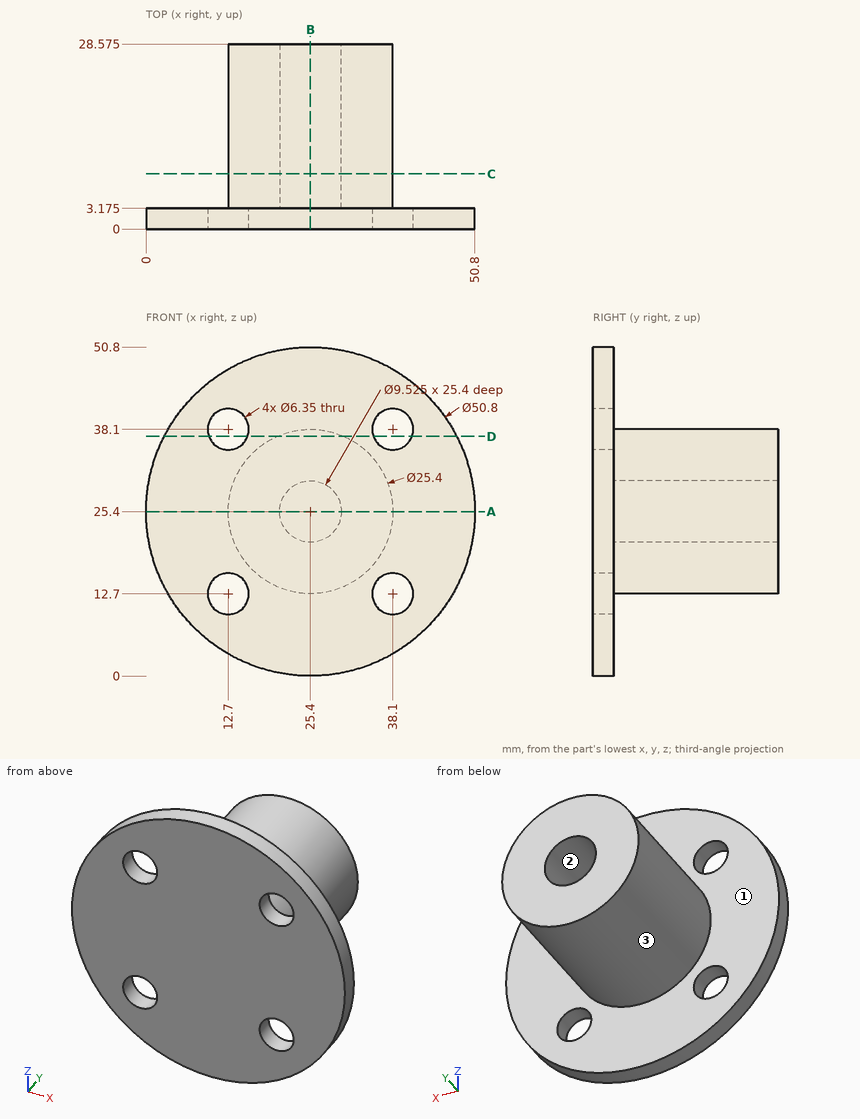
Drawing for the job (mm, zero at the part's lowest x, y, z). Give positions to 0.01 mm unless a question says otherwise; leave off trailing zeros. Order: outer loops, then holes, each group sorted by start corner. A loop starts at its lowest first (then second) coordinate and runs counter-clockwise, first axis right, second up. Notation, with made-up numbers: M -10,14 L 12,14 A17 ccw 12,44 Z; hole C -8,40 d10. An arc over 180 degrees is marked long. Put each result on its own line as item: value.
Item 1: Probe line 1 (X direction, y = 11, z = 25.4); line 2 (Z direction, x = 11, y = 1.5); line 3 (Z direction, x = 12.7, y = 1) (3 decimals). List the from-to ranges inside material, lowest first. Write a range as [from, to].
From the geometry:
line 1: x = [12.7, 20.64], [30.16, 38.1]
line 2: z = [4.48, 10.02], [15.38, 35.42], [40.78, 46.32]
line 3: z = [3.403, 9.525], [15.875, 34.925], [41.275, 47.397]
Item 2: Flat gauge pins, fed straight in: pin 1 Ø4 at (x, z) = (10.5, 33.5) entering from +Y (3 decimals); pin 2 Ø12 at (x, y) = (12.5, 16.5) entering from -Z; pin 3 Ø1 at (x, y) = (17.5, 23.5) entering from +Z. Where does each tip first touch, or does it go through?
From the geometry:
pin 1: stops at y = 3.175
pin 2: stops at z = 14.74
pin 3: stops at z = 35.72
Item 3: Slice it at B-B, the plane x = 25.4. Write the cut outline in (y, z) (1 decimal), plus the area to 3 significant figures.
From the geometry:
outline: M 0,0 L 3.2,0 L 3.2,12.7 L 28.6,12.7 L 28.6,20.6 L 3.2,20.6 L 3.2,30.2 L 28.6,30.2 L 28.6,38.1 L 3.2,38.1 L 3.2,50.8 L 0,50.8 Z
area: 565 mm2
Item 4: Slice it at C-C, the plane y = 8.5. Write the cut outline in (x, z) (1 decimal), plus the area to 3 significant figures.
From the geometry:
outline: C 25.4,25.4 d25.4; hole C 25.4,25.4 d9.5
area: 435 mm2
Item 5: Two-plate mould, pull along X, no slides. Class the marked faces 1, 2 and 3: +X half, -X half, draft (parallel to the pull), parting line (faces both ways), or undercut.
From the geometry:
face 1: draft
face 2: undercut
face 3: parting line
Item 6: Slice it at D-D, the plane z = 37. Write the cut outline in (x, y) (3 decimals), plus the area to 3 significant figures.
From the geometry:
outline: M 2.804,0 L 9.722,0 L 9.722,3.175 L 2.804,3.175 Z; M 15.678,0 L 35.122,0 L 35.122,3.175 L 30.57,3.175 L 30.57,28.575 L 20.23,28.575 L 20.23,3.175 L 15.678,3.175 Z; M 41.078,0 L 47.996,0 L 47.996,3.175 L 41.078,3.175 Z
area: 368 mm2
Item 7: Slice it at A-A, the plane z = 25.4. Write the cut outline in (x, y) (1 decimal), plus the area to 3 significant figures.
From the geometry:
outline: M 0,0 L 50.8,0 L 50.8,3.2 L 38.1,3.2 L 38.1,28.6 L 30.2,28.6 L 30.2,3.2 L 20.6,3.2 L 20.6,28.6 L 12.7,28.6 L 12.7,3.2 L 0,3.2 Z
area: 565 mm2
